from build123d import *

# Parameters (mm, degrees)
F1_DEPTH = 3
F2_DEPTH = 40


with BuildPart() as f1:
    # F0 (on Top) → F1 (new body)
    with BuildSketch(Plane.XY):
        with BuildLine():
            Line((-126.8924768851, 50.456767044), (-145.0232239954, 50.456767044))
            Line((-145.0232239954, 50.456767044), (-146.5232239827, 50.4565720597))
            Line((-146.5232239827, 50.4565720597), (-146.5232239827, 42.9567671074))
            Line((-146.5232239827, 42.9567671074), (-132.4272471595, 42.958404326))
            ThreePointArc((-132.4272471595, 42.958404326), (-129.7719511525, 46.7903220915), (-126.8924768851, 50.456767044))
        make_face()
        Polygon((-146.5232239827, 42.9567671074), (-146.5232239827, 50.4565720597), (-148.02322397, 50.4563770754), (-148.02322397, -49.5432321111), (-146.5232239827, -49.5432321111), (-146.5232239827, -42.0432321745), align=None)
        with BuildLine():
            Line((-145.0102250409, -49.5432321111), (-126.8755409492, -49.5432321111))
            ThreePointArc((-126.8755409492, -49.5432321111), (-129.7580814774, -45.8752925216), (-132.4161980482, -42.0415949559))
            Line((-132.4161980482, -42.0415949559), (-146.5232239827, -42.0432321745))
            Line((-146.5232239827, -42.0432321745), (-146.5232239827, -49.5432321111))
            Line((-146.5232239827, -49.5432321111), (-145.0102250409, -49.5432321111))
        make_face()
        with BuildLine():
            ThreePointArc((-132.4161980482, -42.0415949559), (-145.0167245182, 0.4567674665), (-132.4272471595, 42.958404326))
            Line((-132.4272471595, 42.958404326), (-146.5232239827, 42.9567671074))
            Line((-146.5232239827, 42.9567671074), (-146.5232239827, -42.0432321745))
            Line((-146.5232239827, -42.0432321745), (-132.4161980482, -42.0415949559))
        make_face()
    extrude(amount=-F1_DEPTH)

    # F0 (on Top) → F2 (join)
    with BuildSketch(Plane.XY):
        with BuildLine():
            Line((-126.8924768851, 50.456767044), (-145.0232239954, 50.456767044))
            Line((-145.0232239954, 50.456767044), (-146.5232239827, 50.4565720597))
            Line((-146.5232239827, 50.4565720597), (-146.5232239827, 42.9567671074))
            Line((-146.5232239827, 42.9567671074), (-132.4272471595, 42.958404326))
            ThreePointArc((-132.4272471595, 42.958404326), (-129.7719511525, 46.7903220915), (-126.8924768851, 50.456767044))
        make_face()
        with BuildLine():
            Line((-145.0102250409, -49.5432321111), (-126.8755409492, -49.5432321111))
            ThreePointArc((-126.8755409492, -49.5432321111), (-129.7580814774, -45.8752925216), (-132.4161980482, -42.0415949559))
            Line((-132.4161980482, -42.0415949559), (-146.5232239827, -42.0432321745))
            Line((-146.5232239827, -42.0432321745), (-146.5232239827, -49.5432321111))
            Line((-146.5232239827, -49.5432321111), (-145.0102250409, -49.5432321111))
        make_face()
        Polygon((-146.5232239827, 42.9567671074), (-146.5232239827, 50.4565720597), (-148.02322397, 50.4563770754), (-148.02322397, -49.5432321111), (-146.5232239827, -49.5432321111), (-146.5232239827, -42.0432321745), align=None)
    extrude(amount=F2_DEPTH)


solid = f1.part
Verification items for the finished model (mm, model axes). A direction names the side the tool comes from. Give positions to 0.01 mm unless a question says otherwise; leave off trailing zeros. Loops run counter-clockwise (first coordinate to the right, second up) from the corner with the lowest first, then second, coordinate; pieces in that order, holes last.
1) Sectioned sample at B-B, the plane z = 36. Enter the section's corners in (x, y).
2) Sectioned sample at C-C, the plane y = 0.5. Enter the section's corners in (x, z).
3) Sectioned sample at D-D, the plane x = -144. Enter the section's corners in (y, z).
4) Thickness scan on line 1 along Y through (x, z) = (-138.25, 32); line 2 along X through (y, z) = (43, 29); line 3 along X through (y, z) = (22, 37.5). Record the ranges inside material, lowest first.
5) Depth check by flat-ended pin: pin 1 Ø12 at (x, y) = (-136, -17.5) entering from +Z; pin 2 Ø2 at (x, y) = (-143, 40) entering from +Z; pin 3 Ø3 at (y, z) = (34.5, 23) entering from +X. Enter the tip coordinate at first touch or a pass-through.
6) Sectioned sample at A-A, the plane x = -135. Enter the section's corners in (y, z), then the cut area to 3 significant figures.
7) Set-up check for faces 1 (the flat face through (-138, -49.543, 18)), 2 (the flat face through (-146, 1, 0)): record each of +Z, -Z, +X, -X, +Y, -Y from which the full face is reachable in a straight line by a thin tool's end or side.
Answers:
1. outline: (-148.02, -49.54) - (-126.88, -49.54) arc R78 cw to (-132.42, -42.04) - (-146.52, -42.04) - (-146.52, 42.96) - (-132.43, 42.96) arc R78 cw to (-126.89, 50.46) - (-145.02, 50.46) - (-148.02, 50.46) - close
2. outline: (-148.02, -3) - (-145.02, -3) - (-145.02, 0) - (-146.52, 0) - (-146.52, 40) - (-148.02, 40) - close
3. outline: (-49.54, -3) - (-12.09, -3) - (-12.09, 0) - (-42.04, 0) - (-42.04, 40) - (-49.54, 40) - close; (13.02, -3) - (50.46, -3) - (50.46, 40) - (42.96, 40) - (42.96, 0) - (13.02, 0) - close
4. line 1: y = -49.54 to -42.04, 42.96 to 50.46
4. line 2: x = -148.02 to -132.4
4. line 3: x = -148.02 to -146.52
5. pin 1: passes through
5. pin 2: stops at z = 0
5. pin 3: stops at x = -146.52
6. outline: (-49.54, -3) - (-37.77, -3) - (-37.77, 0) - (-42.04, 0) - (-42.04, 40) - (-49.54, 40) - close; (38.71, -3) - (50.46, -3) - (50.46, 40) - (42.96, 40) - (42.96, 0) - (38.71, 0) - close
6. area: 671 mm2
7. face 1: +Z, -Z, +X, -X, -Y
7. face 2: +Z, +X
